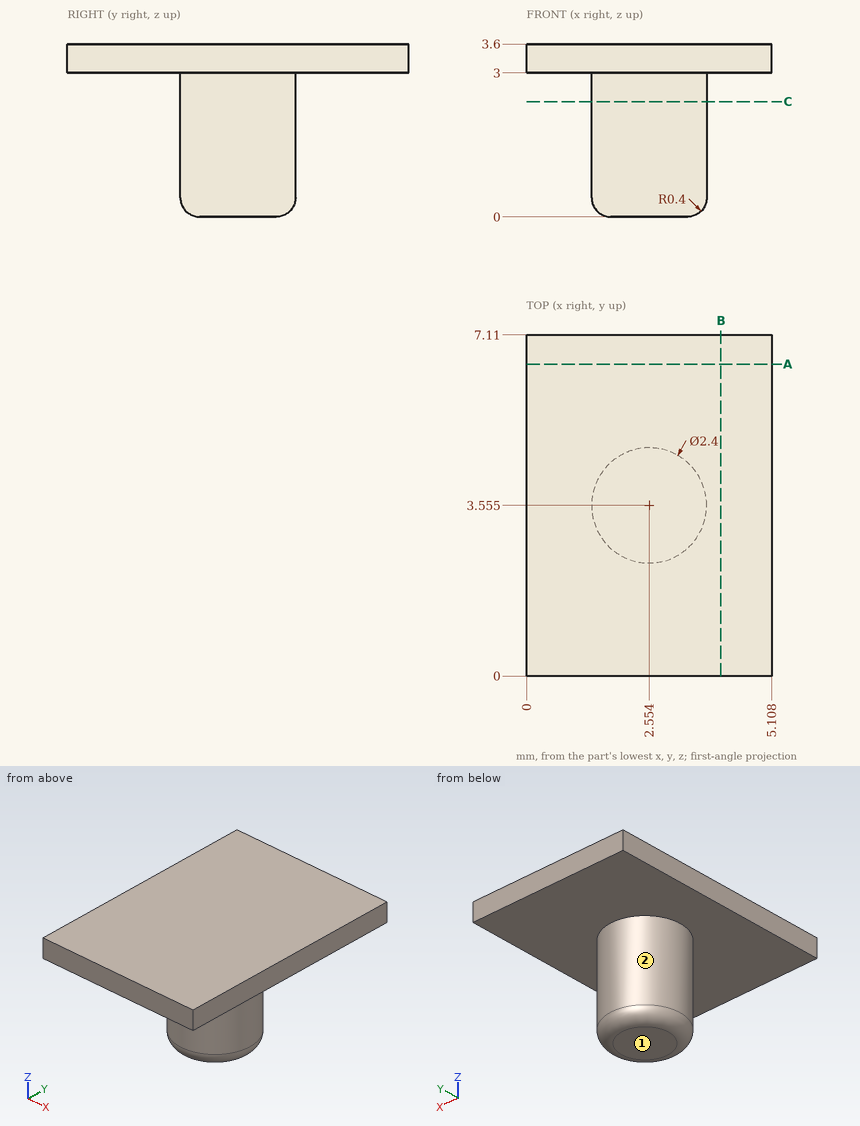
Geometry: see drawing. Coordinates: mm, zero at the bounding-box minimum. A direction names the side the tool comes from. Coordinates: 2 decimals unless noted, no trailing zeros. Loops run counter-clockwise (first coordinate to the right, second up) from the corner with the lowest first, then second, coordinate; pieces in that order, holes last. Notation, with made-up numbers: (-18.5, 35.5) - (-0.5, 35.5) arc R18 ccw to (-0.5, 64.5) - close; hole circle Ø10 at (71, -6.5). An arc over 180 degrees is marked (long way). Return JSON: item names as keys, results as strings.
Q1. Section C-C, the plane z = 2.4. Return loops of the section in (x, y) (3 decimals).
Results:
{"outline": "circle Ø2.4 at (2.554, 3.555)"}
Q2. Contact query for a flat-ended pin moving along its axis: P1, Ø1.5, axis at y = 6.5, z = 1.5, coming from the +X side. Output: stop coordinate, or through.
Results:
{"P1": "through"}
Q3. Access query for the marked faces 1 and 2. Directions: +Z, -Z, +X, -X, +Y, -Y. A direction counts if a zero-diameter tool reaches every point of the face in a straight line with its end or side. Return the directions, or none.
Results:
{"face 1": "-Z, +X, -X, +Y, -Y", "face 2": "-Z"}
Q4. Section A-A, the plane y = 6.5. Return loops of the section in (x, z).
Results:
{"outline": "(0, 3) - (5.11, 3) - (5.11, 3.6) - (0, 3.6) - close"}
Q5. Section B-B, the plane x = 4.05. Return loops of the section in (y, z), plus the area to 3 significant figures.
Results:
{"outline": "(0, 3) - (7.11, 3) - (7.11, 3.6) - (0, 3.6) - close", "area": "4.27 mm2"}
Q6. Material intervals for line 1 along Z through (x, y) = (4.55, 5); line 2 along X through (y, z) = (3.5, 0.75); line 3 along Y through (x, z) = (3.55, 2.9), sorted ascending.
Results:
{"line 1": "3 to 3.6", "line 2": "1.36 to 3.75", "line 3": "2.89 to 4.22"}
